```python
from build123d import *

# Parameters (mm, degrees)
SKETCH1_R           = 1.5
SKETCH1_R_2         = 1.7
BOSS_EXTRUDE1_DEPTH = 4
CUT_EXTRUDE1_DEPTH  = 5
FILLET1_R           = 1


with BuildPart() as part:
    # Sketch1 → Boss-Extrude1 (new body)
    with BuildSketch(Plane.XY):
        with BuildLine():
            Line((-17.976190476, -2.545770461), (17.023809524, -2.545770461))
            ThreePointArc((17.023809524, -2.545770461), (21.971428708, 1.732381628), (18.452380952, 7.245803777))
            Line((18.452380952, 7.245803777), (5.595238095, 11.079063167))
            ThreePointArc((5.595238095, 11.079063167), (3.465102786, 11.443404154), (1.30952381, 11.28945588))
            Line((1.30952381, 11.28945588), (-18.928571429, 7.362688617))
            ThreePointArc((-18.928571429, 7.362688617), (-22.953252631, 1.975844438), (-17.976190476, -2.545770461))
        make_face()
        with Locations((-17.976190476, 2.454229539)):
            Circle(SKETCH1_R, mode=Mode.SUBTRACT)
        with Locations((3.023809524, 2.454229539)):
            Circle(SKETCH1_R_2, mode=Mode.SUBTRACT)
    extrude(amount=BOSS_EXTRUDE1_DEPTH)

    # Sketch2 → Cut-Extrude1 (cut, through all)
    with BuildSketch(Plane.XY.offset(4)):
        with BuildLine():
            Line((-1.835195666, -8.126804745), (2.106929637, -8.126804745))
            ThreePointArc((2.106929637, -8.126804745), (4.059880255, -2.995686673), (4.723809524, 2.454229539))
            ThreePointArc((4.723809524, 2.454229539), (3.023809524, 4.154229539), (1.323809524, 2.454229539))
            ThreePointArc((1.323809524, 2.454229539), (0.517202937, -3.067038438), (-1.835195666, -8.126804745))
        make_face()
    extrude(amount=-CUT_EXTRUDE1_DEPTH, mode=Mode.SUBTRACT)

    # Fillet1
    fillet1_edges = [part.edges().sort_by_distance(p)[0] for p in [
        (4.166302608, -2.545770461, 2),
        (0.664893183, -2.545770461, 2),
    ]]
    fillet(fillet1_edges, radius=FILLET1_R)


solid = part.part
```
CAD build for the part. Positions are in the model's coordinates, mm. A direction names the side the tool comes from. Give positions to 0.01 mm unless a question says otherwise; leave off trailing zeros. Loops run counter-clockwise (first coordinate to the right, second up) from the corner with the lowest first, then second, coordinate; pieces in that order, holes last. Notation, with made-up numbers: (21.25, -30) - (71.25, -30) arc R22 ccw to (71.25, -14) - close; hole circle Ø2 at (-37.75, 55). An arc over 180 degrees is marked (long way). Put each result on its own line as item: value.
Q1. Tool access for faces 5 (the face through (0.5, -2.33, 2.03)), 6 (the face through (-1, 3, 4)), 7 (the face through (3.061, 4.154, 1.972)): list every direction of +Z, -Z, +X, -X, +Y, -Y with a clear straight run to the whole face (end or side of a thin tool).
Filled in:
face 5: +Z, -Z, -Y
face 6: +Z, +X, -X, +Y, -Y
face 7: +Z, -Z
Q2. Flat gauge pin, fed straight in: pin 1 (2.5 mm diameter, centred on x = -17.98, y = 2.45, fed in from +Z). Where does the tip first touch, or does it go through?
Filled in:
pin 1: passes through
Q3. Slice it at D-D (y = 6.75). Give the cut face in (x, z), plus the area to 3 significant figures.
Filled in:
outline: (-20.53, 0) - (19.58, 0) - (19.58, 4) - (-20.53, 4) - close
area: 160 mm²
Q4. Slice it at A-A (z = 3.6). Give the cut face in (x, y), plus the area to 3 significant figures.
Filled in:
outline: (-18.93, 7.36) arc R5 ccw to (-17.98, -2.55) - (-0.12, -2.55) arc R1 ccw to (0.86, -1.76) arc R19.3 ccw to (1.32, 2.45) arc R1.7 cw to (4.72, 2.45) arc R22.7 cw to (4.4, -1.38) arc R1 ccw to (5.38, -2.55) - (17.02, -2.55) arc R5 ccw to (18.45, 7.25) - (5.6, 11.08) arc R9 ccw to (1.31, 11.29) - close; hole circle Ø3 at (-17.98, 2.45)
area: 476 mm²
Q5. Slice it at C-C (x = 19). Give the cut face in (y, z), plus the area to 3 significant figures.
Filled in:
outline: (-2.14, 0) - (7.05, 0) - (7.05, 4) - (-2.14, 4) - close
area: 36.7 mm²
Q6. Probe line 1 along X through (y, z) = (2, 3.45); line 2 along X through (y, z) = (3.75, 0.3); line 3 along X through (y, z) = (-1.25, 0.9) (3 decimals). List the from-to ranges inside material, lowest first.
Filled in:
line 1: x = -22.96 to -19.41, -16.55 to 1.32, 4.72 to 22
line 2: x = -22.81 to -18.73, -17.22 to 1.92, 4.12 to 21.85
line 3: x = -21.335 to 0.965, 4.42 to 20.382
Q7. Mould opens along X. For faces 1 (the face through (-16.545, 2.905, 1.972)), 2 (the face through (-1, 3, 0)), 3 (the face through (3.5, 11.44, 1.97)), 4 (the face through (1.21, 0.36, 2.03)) say: pulls with the +X half, pulls with the -X half, needs draft (parallel to the pull), parting line crosses it, or undercut.
Filled in:
face 1: undercut
face 2: needs draft
face 3: parting line crosses it
face 4: undercut
Q8. Slice it at B-B (y = 0). Give the cut face in (x, z), plus the area to 3 significant figures.
Filled in:
outline: (-22.33, 0) - (1.17, 0) - (1.17, 4) - (-22.33, 4) - close; (4.59, 0) - (21.38, 0) - (21.38, 4) - (4.59, 4) - close
area: 161 mm²
